Could you check a few things on this model? Use its own coordinates, in mm. A direction names the side the tool comes from. Round coordinates to 2 decimals unless told otherwise and drop trailing zeros. Write each loop counter-clockwise with the first axis right and the second up, starting at its lowest first coordinate (ties: lowest second). Pieces come first, ordered by that corner, then holes. Notation, with made-up numbers: (-17, 16.25) -> (-2, 16.25) arc R23 cw to (-2, 29.25) -> close; hole circle Ø1 at (52.25, 65.5). An arc over 180 degrees is marked (long way). Answer in a Markdown table with one row per item. Add a question column.
```python
from build123d import *

# Parameters (mm, degrees)
SKETCH_1_R          = 27
SKETCH_1_R_2        = 5
EXTRUDE_1_DEPTH     = 7
SKETCH_4_R          = 21
CUT_EXTRUDE_1_DEPTH = 2
SKETCH_5_R          = 21
SKETCH_5_R_2        = 7
CUT_EXTRUDE_2_DEPTH = 3


with BuildPart() as part:
    # 草图1 → 凸台-拉伸1 (new, symmetric)
    with BuildSketch(Plane.XY):
        Circle(SKETCH_1_R)
        Circle(SKETCH_1_R_2, mode=Mode.SUBTRACT)
    extrude(amount=EXTRUDE_1_DEPTH, both=True)

    # 草图2 → 切除-旋转1 (revolve, cut)
    with BuildSketch(Plane(origin=(0, 0, 0), x_dir=(0, 0, -1), z_dir=(1, 0, 0))):
        with BuildLine():
            Line((-6.5814e-13, 27), (-7, 27))
            Line((-7, 27), (-7, 26.076809620810586))
            ThreePointArc((-7.0000000000000195, 26.07680962081059), (-3.530307368921202, 26.768207446165324), (-6.5782e-13, 27))
        make_face()
        with BuildLine():
            Line((7, 27), (-6.5814e-13, 27))
            ThreePointArc((-6.5782e-13, 27), (3.5303073689204805, 26.76820744616542), (6.999999999999878, 26.076809620810625))
            Line((7, 26.076809620810657), (7, 27))
        make_face()
    revolve(axis=Axis((0, 0, -7), (0, 0, 1)), mode=Mode.SUBTRACT)

    # 草图4 → 切除-拉伸1 (cut)
    with BuildSketch(Plane.XY.offset(7)):
        Circle(SKETCH_4_R)
    cut_extrude_1 = extrude(amount=-CUT_EXTRUDE_1_DEPTH, mode=Mode.SUBTRACT)

    # 草图5 → 切除-拉伸2 (cut)
    with BuildSketch(Plane.XY.offset(5)):
        Circle(SKETCH_5_R)
        Circle(SKETCH_5_R_2, mode=Mode.SUBTRACT)
    cut_extrude_2 = extrude(amount=-CUT_EXTRUDE_2_DEPTH, mode=Mode.SUBTRACT)

    # 镜向1: 切除-拉伸1, 切除-拉伸2 across plane
    add(cut_extrude_1.mirror(Plane.XY), mode=Mode.SUBTRACT)
    add(cut_extrude_2.mirror(Plane.XY), mode=Mode.SUBTRACT)


solid = part.part
```
(1) For P1, Ø1, axis at x = -1, y = -14.5, coming from the +Z side; P2, Ø5, axis at x = -14.5, z = -0.5, coming from the +Y side; P3, Ø8, axis at y = 13, z = -5, coming from the +X side, each with a flat end and sliding along its axis, tell me the tip position at first contact or that it passes through.
(2) Suppose I cut it at D-D, the plane x = -13.5. Please give me the cut outline in (y, z).
(3) Suppose I cut it at A-A, the plane y = 0. Please give me the cut outline in (x, z).
(4) If we mould it in two halves opening along Y, with no side actions, what happens to faces 1 (the face through (9, 0, -2)), 2 (the face through (-2, 5, -5)), 3 (the face through (-18, 12, 7))? For each: pulls with the +Y half, pulls with the -Y half, needs draft (parallel to the pull), parting line crosses it, or undercut.
(5) I need wall thicknesses on L1, parallel to Y at x = 0, z = -0.5; L2, parallel to Y at x = -1.5, z = -3.25; L3, parallel to Y at x = -4.5, z = 2.5. Which ranges of each line are inside material? Lowest first, please.
(6) Suppose I cut it at C-C, the plane z = 2.75. Please give me the cut outline in (x, y), then the cut area to 3 significant figures.
(7) On a 3-axis mill with a long thin cutter (end or side, diameter ignored), from which of +Z, -Z, +X, -X, +Y, -Y can I reach the whole of each face in a straight line? I mean faces 4 (the face through (20.03, 6.31, -4.54)), 5 (the face through (-18, 12, -7)), 6 (the face through (9, 0, 2)). Say none if no direction works.
Response:
| question | item | result |
|---|---|---|
| 1 | P1 | z = 2 |
| 1 | P2 | y = 24.18 |
| 1 | P3 | x = 25.11 |
| 2 | outline | (-22.31, -7) -> (-16.09, -7) -> (-16.09, -2) -> (16.09, -2) -> (16.09, -7) -> (22.31, -7) arc R23.38 ccw to (22.31, 7) -> (16.09, 7) -> (16.09, 2) -> (-16.09, 2) -> (-16.09, 7) -> (-22.31, 7) arc R23.38 ccw to start |
| 3 | outline | (-26.08, -7) -> (-21, -7) -> (-21, -2) -> (-7, -2) -> (-7, -5) -> (-5, -5) -> (-5, 5) -> (-7, 5) -> (-7, 2) -> (-21, 2) -> (-21, 7) -> (-26.08, 7) arc R27 ccw to start; (5, -5) -> (7, -5) -> (7, -2) -> (21, -2) -> (21, -7) -> (26.08, -7) arc R27 ccw to (26.08, 7) -> (21, 7) -> (21, 2) -> (7, 2) -> (7, 5) -> (5, 5) -> close |
| 4 | face 1 | undercut |
| 4 | face 2 | undercut |
| 4 | face 3 | needs draft |
| 5 | L1 | -27 to -5, 5 to 27 |
| 5 | L2 | -26.76 to -20.95, -6.84 to -4.77, 4.77 to 6.84, 20.95 to 26.76 |
| 5 | L3 | -26.5 to -20.51, -5.36 to -2.18, 2.18 to 5.36, 20.51 to 26.5 |
| 6 | outline | circle Ø53.72 at (0, 0); circle Ø14 at (0, 0); hole circle Ø42 at (0, 0); hole circle Ø10 at (0, 0) |
| 6 | area | 956 mm² |
| 7 | face 4 | -Z |
| 7 | face 5 | -Z, +X, -X, +Y, -Y |
| 7 | face 6 | +Z |
